Verification items for the finished model (mm, model axes). A direction names the side the tool comes from. Coordinates: 2 decimals unless noted, no trailing zeros. Order: outer loops, then holes, each group sorted by start corner. A loop starts at its lowest first (then second) coordinate and runs counter-clockwise, first axis right, second up.
Q1. Set-up check for faces 1 (the flat face through (33.604, -127, 41)), 2 (the cylindrical face through (-71.535, 92.168, -4.684)), 3 (the flat face through (-33.604, -126, 41)), 4 (the cylindrical face through (24.19, -126.26, 73.18)), 5 (the cylindrical face through (-23.68, -126.74, 9.41)): record each of +Z, -Z, +X, -X, +Y, -Y from which the full face is reachable in a straight line by a thin tool's end or side.
Q2. Cross-section at C-C, the plane z = -4. Record the boundary of the cut face in (x, y).
Q3. Cross-section at B-B, the plane x = 48. Record the boundary of the cut face in (y, z).
Q4. Thickness scan on line 1 (Y direction, x = -80, z = 5); line 2 (Y direction, x = 219, z = 8); line 3 (X direction, y = 107, z = 6). Record the ranges inside material, lowest first.
Q5. Cross-section at A-A, the plane y = 67. Record the boundary of the cut face in (x, z).
Q6. Draft check along Y on faces 6 (the cylindrical face through (-88.99, 117.62, 34.53)), 7 (the flat face through (-57, -109.7, 41)), 8 (the cylindrical face through (198.81, -85.56, -4.68)). Enter one of: pulls with the +Y half, pulls with the -Y half, needs draft (parallel to the pull), parting line crosses it, or undercut.
Q7. Cross-section at D-D, the plane z = 20. Record the boundary of the cut face in (x, y).
Q8. Depth check by flat-ended pin: P1, Ø12, axis at x = 189, y = -23, coming from the -Z side; P2, Ø5, axis at y = -124, z = 39.5, coming from the -X side; P3, Ø8.5, axis at y = -120.5, z = 41.5, coming from the +X side. Enter the tip coordinate at first touch or a pass-through.
from build123d import *

# Parameters (mm, degrees)
F1_DEPTH = 83.1
F2_R     = 8.2679972053
F3_DEPTH = 9.5
F4_R     = 15
F5_R     = 33
F7_D     = 4.4
F7_DEPTH = 12
F7_TIP   = 1.3218933619


with BuildPart() as f1:
    # F0 (on Top) → F1 (new body)
    with BuildSketch(Plane.XY):
        Polygon((232.5, 121.9), (-93.5, 121.9), (-93.5, -109.7), (-33.6043722928, -109.7), (-33.6043722928, -143.3), (33.6043722928, -143.3), (33.6043722928, -109.7), (232.5, -109.7), align=None)
    extrude(amount=F1_DEPTH)

    # F2 (on face) → F3 (join)
    with BuildSketch(Plane(origin=(0, 0, 0), x_dir=(1, 0, 0), z_dir=(0, 0, -1))):
        with Locations((-65.4409214878, 88.7281829967)):
            Circle(F2_R)
        with Locations((-65.4409214878, -97.7562729967)):
            Circle(F2_R)
        with Locations((191.1744738977, 88.7281829967)):
            Circle(F2_R)
        with Locations((191.1744738977, -97.7562729967)):
            Circle(F2_R)
    extrude(amount=F3_DEPTH)

    # F4
    f4_edges = [f1.edges().sort_by_distance(p)[0] for p in [
        (-93.5, -109.7, 41.55),
        (232.5, -109.7, 41.55),
        (-93.5, 121.9, 41.55),
        (232.5, 121.9, 41.55),
        (69.5, 121.9, 83.1),
        (-93.5, 6.1, 83.1),
        (232.5, 6.1, 83.1),
    ]]
    fillet(f4_edges, radius=F4_R)

    # F5
    f5_edges = [f1.edges().sort_by_distance(p)[0] for p in [
        (-33.604372, -126.5, 83.1),
        (33.604372, -126.5, 83.1),
        (-33.604372, -126.5, 0),
        (33.604372, -126.5, 0),
    ]]
    fillet(f5_edges, radius=F5_R)

    # F7
    with Locations(Plane(origin=(0, 0, 0), x_dir=(1, 0, 0), z_dir=(0, 0, -1))):
        with Locations((-80.5, 51.9), (55, -25), (101, -107), (219, -23)):
            Hole(F7_D / 2, depth=F7_DEPTH)
            with Locations((0, 0, -(F7_DEPTH + F7_TIP / 2))):  # 118° drill point
                Cone(0, F7_D / 2, F7_TIP, mode=Mode.SUBTRACT)


solid = f1.part
Check values:
1. face 1: +Z, -Z, +X, -Y
1. face 2: -Z
1. face 3: +Z, -Z, -X, -Y
1. face 4: +Z, +X, -Y
1. face 5: -Z, -X, -Y
2. outline: circle Ø16.54 at (-65.44, -88.73); circle Ø16.54 at (-65.44, 97.76); circle Ø16.54 at (191.17, -88.73); circle Ø16.54 at (191.17, 97.76)
3. outline: (-109.7, 0) - (121.9, 0) - (121.9, 68.1) arc R15 ccw to (106.9, 83.1) - (-109.7, 83.1) - close
4. line 1: y = -109.62 to -54.04, -49.76 to 121.82
4. line 2: y = -109.62 to 20.8, 25.2 to 121.82
4. line 3: x = -93.5 to 98.8, 103.2 to 232.5
5. outline: (-93.5, 0) - (232.5, 0) - (232.5, 68.1) arc R15 ccw to (217.5, 83.1) - (-78.5, 83.1) arc R15 ccw to (-93.5, 68.1) - close
6. face 6: pulls with the +Y half
6. face 7: pulls with the -Y half
6. face 8: undercut
7. outline: (-93.5, -94.7) arc R15 ccw to (-78.5, -109.7) - (-30.94, -109.7) - (-30.94, -143.3) - (30.94, -143.3) - (30.94, -109.7) - (217.5, -109.7) arc R15 ccw to (232.5, -94.7) - (232.5, 106.9) arc R15 ccw to (217.5, 121.9) - (-78.5, 121.9) arc R15 ccw to (-93.5, 106.9) - close
8. P1: stops at z = 0
8. P2: stops at x = -33.6
8. P3: stops at x = 33.6
